Check sheet for the modelled part. Datum: model origin and axes. Units: mm. A direction names the side the tool comes from. Round coordinates to 2 decimals unless told otherwise and drop trailing zeros. Write each loop counter-clockwise with the first axis right and the second up, starting at its lowest first coordinate (ties: lowest second). Pieces come first, ordered by that corner, then holes.
Item 1: Release check for a two-part mould opening along X. For faces 3 (the cylindrical face through (-11.291, -1.479, 5.693)), 4 (the flat face through (-12, 0, 5)), 5 (the flat face through (-13, -3, 0)), 6 (the cylindrical face through (-26.77, -0.04, -26.7)) record: +X half, -X half, draft (parallel to the pull), parting line (faces both ways), or undercut.
Item 2: Cross-section at C-C on y = -0.9. Count the separate pieces of the cut face and the enclosed holes in it, plus the area to 3 significant figures.
Item 3: Go/stop test with flat-tipped pins: pin 1 Ø5 at (x, z) = (-0.5, -13.5) entering from +Y; pin 2 Ø1.8 at (x, z) = (-11.5, 6.5) entering from +Y. Record where each tip stops, or that it passes through.
Item 4: Tool access check on faces 1 (the cylindrical face through (20.973, -0.042, 23.684)), 2 (the flat face through (1.3, 0, -12.7)). Record the directions out of +Z, -Z, +X, -X, +Y, -Y that give a thin tool (end or side, any length) a straight path to the whole face; none if there is none.
Item 5: Material ranges on line 1 (Z direction, x = -23.57, y = -0.8); line 2 (Z direction, x = 0, y = -2.2); line 3 (Z direction, x = -22, y = 0.35), recorded low to high.
Item 6: Cross-section at A-A on z = 0. Enter the section's corners in (x, y).
Item 7: Cross-section at B-B on x = -5. Enter the section's corners in (y, z), plus the area to 3 significant figures.
Item 8: Cross-section at D-D on z = 14. Enter the section's corners in (x, y).
from build123d import *

# Parameters (mm, degrees)
SKETCH1_W           = 56.4
SKETCH1_H           = 56.4
BOSS_EXTRUDE1_DEPTH = 3
FILLET1_R           = 5
SKETCH2_R           = 2.6
CUT_EXTRUDE1_DEPTH  = 7
SKETCH4_R           = 10
CUT_EXTRUDE3_DEPTH  = 7
SKETCH5_R           = 1.55
CUT_EXTRUDE4_DEPTH  = 7
SKETCH6_R           = 3
CUT_EXTRUDE5_DEPTH  = 3
CIRPATTERN1_COUNT   = 6


with BuildPart() as part:
    # Sketch1 → Boss-Extrude1 (new body, symmetric)
    with BuildSketch(Plane(origin=(0, 0, 0), x_dir=(1, 0, 0), z_dir=(0, 1, 0))):
        Rectangle(SKETCH1_W, SKETCH1_H)
    extrude(amount=BOSS_EXTRUDE1_DEPTH, both=True)

    # Fillet1
    fillet1_edges = [part.edges().sort_by_distance(p)[0] for p in [
        (28.2, 0, 28.2),
        (-28.2, 0, 28.2),
        (-28.2, 0, -28.2),
        (28.2, 0, -28.2),
    ]]
    fillet(fillet1_edges, radius=FILLET1_R)

    # Sketch2 → Cut-Extrude1 (cut, through all)
    with BuildSketch(Plane.XZ.offset(3)):
        with Locations((-23.57, 23.57)):
            Circle(SKETCH2_R)
        with Locations((23.57, 23.57)):
            Circle(SKETCH2_R)
        with Locations((23.57, -23.57)):
            Circle(SKETCH2_R)
        with Locations((-23.57, -23.57)):
            Circle(SKETCH2_R)
    extrude(amount=-CUT_EXTRUDE1_DEPTH, mode=Mode.SUBTRACT)

    # Sketch4 → Cut-Extrude3 (cut, through all)
    with BuildSketch(Plane.XZ.offset(3)):
        Circle(SKETCH4_R)
    extrude(amount=-CUT_EXTRUDE3_DEPTH, mode=Mode.SUBTRACT)

    # Sketch5 → Cut-Extrude4 (cut, through all)
    with BuildSketch(Plane(origin=(0, 3, 0), x_dir=(1, 0, 0), z_dir=(0, 1, 0))):
        with Locations((0, 14)):
            Circle(SKETCH5_R)
    cut_extrude4 = extrude(amount=-CUT_EXTRUDE4_DEPTH, mode=Mode.SUBTRACT)

    # Sketch6 → Cut-Extrude5 (cut)
    with BuildSketch(Plane(origin=(0, 3, 0), x_dir=(1, 0, 0), z_dir=(0, 1, 0))):
        with Locations((0, 14)):
            Circle(SKETCH6_R)
    cut_extrude5 = extrude(amount=-CUT_EXTRUDE5_DEPTH, mode=Mode.SUBTRACT)

    # CirPattern1: Cut-Extrude4, Cut-Extrude5 ×6 about axis
    cirpattern1_axis = Axis((0, 0, 0), (0, 1, 0))
    for i in range(1, CIRPATTERN1_COUNT):
        add(cut_extrude4.rotate(cirpattern1_axis, i * 360 / CIRPATTERN1_COUNT), mode=Mode.SUBTRACT)
        add(cut_extrude5.rotate(cirpattern1_axis, i * 360 / CIRPATTERN1_COUNT), mode=Mode.SUBTRACT)


solid = part.part
Response values:
1. face 3: undercut
1. face 4: undercut
1. face 5: draft
1. face 6: -X half
2. separate pieces: 1
2. enclosed holes: 11
2. area: 2,720 mm2
3. pin 1: stops at y = 3
3. pin 2: stops at y = 0
4. face 1: +Y, -Y
4. face 2: +Y
5. line 1: z = -28.19 to -26.17, -20.97 to 20.97, 26.17 to 28.19
5. line 2: z = -28.2 to -15.55, -12.45 to -10, 10 to 12.45, 15.55 to 28.2
5. line 3: z = -28.2 to -25.64, -21.5 to 21.5, 25.64 to 28.2
6. outline: (-28.2, -3) - (-10, -3) - (-10, 3) - (-28.2, 3) - close; (10, -3) - (28.2, -3) - (28.2, 3) - (10, 3) - close
7. outline: (-3, -28.2) - (3, -28.2) - (3, -8.66) - (-3, -8.66) - close; (-3, 8.66) - (3, 8.66) - (3, 28.2) - (-3, 28.2) - close
7. area: 234 mm2
8. outline: (-28.2, -3) - (-1.55, -3) - (-1.55, 0) - (-3, 0) - (-3, 3) - (-28.2, 3) - close; (1.55, -3) - (28.2, -3) - (28.2, 3) - (3, 3) - (3, 0) - (1.55, 0) - close
